The model under review builds one solid part; all positions refer to its coordinate system, in mm. Coordinates: 2 decimals unless noted, no trailing zeros. Write each loop counter-clockwise with the first axis right and the second up, starting at its lowest first coordinate (ties: lowest second). Pieces come first, ordered by that corner, then holes.
```python
from build123d import *

# Parameters (mm, degrees)
F0_W     = 22.225
F0_H     = 22.225
F1_DEPTH = 11.938
F2_R     = 1.5875
F3_DEPTH = 3.175


with BuildPart() as f1:
    # F0 (on Top) → F1 (new body)
    with BuildSketch(Plane.XY):
        with Locations((-10.368031, 17.720491)):
            Rectangle(F0_W, F0_H)
    extrude(amount=F1_DEPTH)

    # F2 (on face) → F3 (join)
    with BuildSketch(Plane(origin=(-21.480531, 0, 0), x_dir=(0, -1, 0), z_dir=(-1, 0, 0))):
        with Locations((-23.635626, 5.858807)):
            Circle(F2_R)
    extrude(amount=F3_DEPTH)


solid = f1.part
```
Item 1: Take a section at A-A, the plane z = 7. Write out the cut boundary in (x, y), plus the area to 3 significant figures.
Solved:
outline: (-24.66, 22.53) - (-21.48, 22.53) - (-21.48, 6.61) - (0.74, 6.61) - (0.74, 28.83) - (-21.48, 28.83) - (-21.48, 24.74) - (-24.66, 24.74) - close
area: 501 mm2
Item 2: Take a section at C-C, the plane z = 1.25. Write out the cut boundary in (x, y), plus the area to 3 significant figures.
Solved:
outline: (-21.48, 6.61) - (0.74, 6.61) - (0.74, 28.83) - (-21.48, 28.83) - close
area: 494 mm2
Item 3: For pin 1 (5 mm diameter, centred on y = 11.5, z = 6.5, fed in from -X), flat-tipped, find the tip position at first contact; note if it passes through.
Solved:
pin 1: stops at x = -21.48
Item 4: Take a section at D-D, the plane x = -22.5. Write out the cut boundary in (y, z) (1 decimal), plus the area to 3 significant figures.
Solved:
outline: circle Ø3.2 at (23.6, 5.9)
area: 7.92 mm2
Item 5: Take a section at B-B, the plane y = 24. Write out the cut boundary in (x, z).
Solved:
outline: (-24.66, 4.31) - (-21.48, 4.31) - (-21.48, 0) - (0.74, 0) - (0.74, 11.94) - (-21.48, 11.94) - (-21.48, 7.4) - (-24.66, 7.4) - close
Item 6: To check wall thickness, follow line 1 along X through (y, z) = (9.5, 2.75). State the ranges of the line that lie inside material, in increasing order.
Solved:
line 1: x = -21.48 to 0.74
Item 7: Mouldability with a two-part tool opening along Y and no side actions: class faces 1 (the face through (-11, 28.833, 6)), 2 (the face through (-21.481, 18, 6)), 3 (the face through (-23.05, 22.17, 5.25)) as pulls with the +Y half, pulls with the -Y half, needs draft (parallel to the pull), parting line crosses it, or undercut.
Solved:
face 1: pulls with the +Y half
face 2: needs draft
face 3: parting line crosses it
